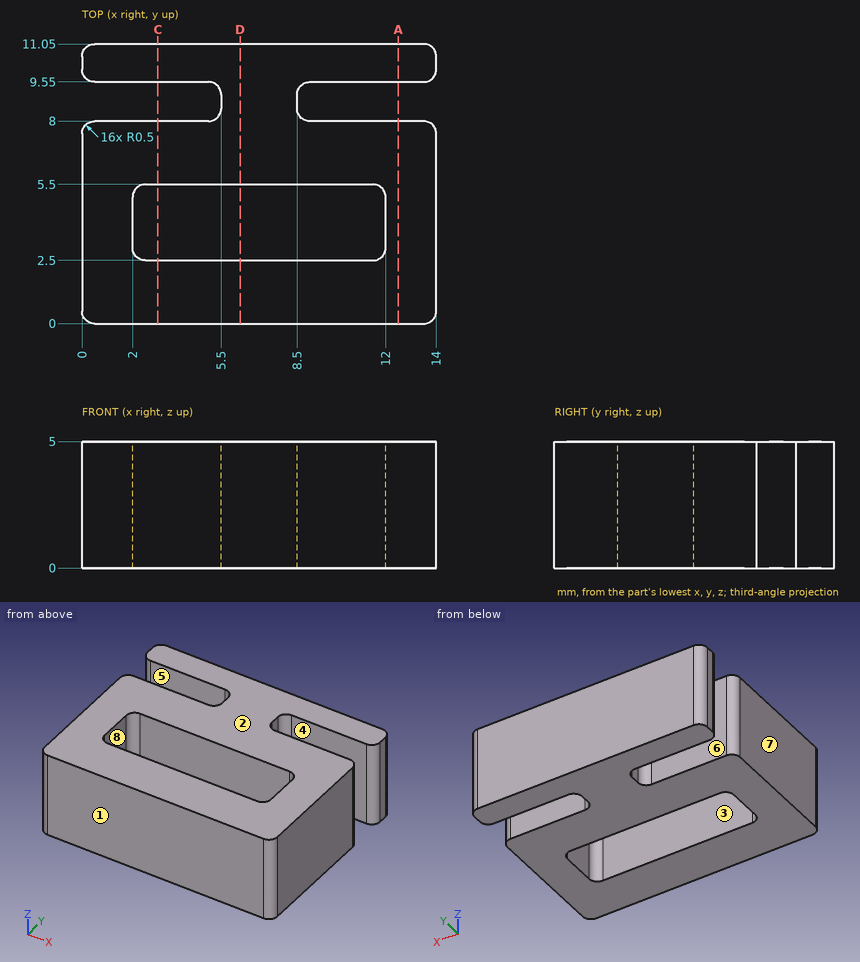
Geometry: see drawing. Coordinates: mm, zero at the bounding-box minimum. A direction names the side the tool comes from. Round coordinates to 2 decimals unless told otherwise and drop trailing zeros. Write each loop counter-clockwise with the first axis right and the second up, starting at its lowest first coordinate (ties: lowest second). Pieces come first, ordered by that corner, then holes. Notation, with made-up numbers: M 11.5,-26.75 L 57.5,-26.75 A32 cw 57.5,9.25 Z; hole C 70.5,4.25 d6. An arc over 180 degrees is marked long. Answer in a Markdown table with one row per item. Add a question column.
(1) Draft query along X for the marked faces 6, 7 and 8. Return one class per face: pulls with the +X half, pulls with the -X half, needs draft (parallel to the pull), parting line crosses it, or undercut.
(2) Ray query, L1, parallel to Y at x = 3.5, z = 0.45; L2, parallel to X at y = 3.75, z = 1.95. Return the intervals inside material, ascending.
(3) Contact query for a flat-ended pin moving along its axis: pin 1 (0.6 mm diameter, centred on y = 9, z = 3, fed in from +X). Output: stop coordinate, or through.
(4) Reachability of the marked faces 1, 2, 3, 4 and 5 from +Z, -Z, +X, -X, +Y, -Y: full face, straight path, thin tool, end or side. Return the list, or none.
(5) Cut plane A-A, the plane x = 12.5. Return the cut outline in (y, z).
(6) Cut plane D-D, the plane x = 6.25. Return the cut outline in (y, z).
(7) Cut plane C-C, the plane x = 3. Return the cut outline in (y, z).
Established:
| question | item | result |
|---|---|---|
| 1 | face 6 | needs draft |
| 1 | face 7 | pulls with the -X half |
| 1 | face 8 | undercut |
| 2 | L1 | 0 to 2.5, 5.5 to 8, 9.55 to 11.05 |
| 2 | L2 | 0 to 2, 12 to 14 |
| 3 | pin 1 | x = 8.57 |
| 4 | face 1 | +Z, -Z, +X, -X, -Y |
| 4 | face 2 | +Z, +X, -X, +Y, -Y |
| 4 | face 3 | +Z, -Z |
| 4 | face 4 | +Z, -Z, +X |
| 4 | face 5 | +Z, -Z, -X |
| 5 | outline | M 0,0 L 8,0 L 8,5 L 0,5 Z; M 9.55,0 L 11.05,0 L 11.05,5 L 9.55,5 Z |
| 6 | outline | M 0,0 L 2.5,0 L 2.5,5 L 0,5 Z; M 5.5,0 L 11.05,0 L 11.05,5 L 5.5,5 Z |
| 7 | outline | M 0,0 L 2.5,0 L 2.5,5 L 0,5 Z; M 5.5,0 L 8,0 L 8,5 L 5.5,5 Z; M 9.55,0 L 11.05,0 L 11.05,5 L 9.55,5 Z |
